Part model, mm, in its own coordinate system. Face numbers are marked on the shaded views. A direction names the side the tool comes from. Coordinates: 2 decimals unless noted, no trailing zeros. Order: outer loops, then holes, each group sorted by start corner. A loop starts at its lowest first (then second) coordinate and runs counter-clockwise, first axis right, second up.
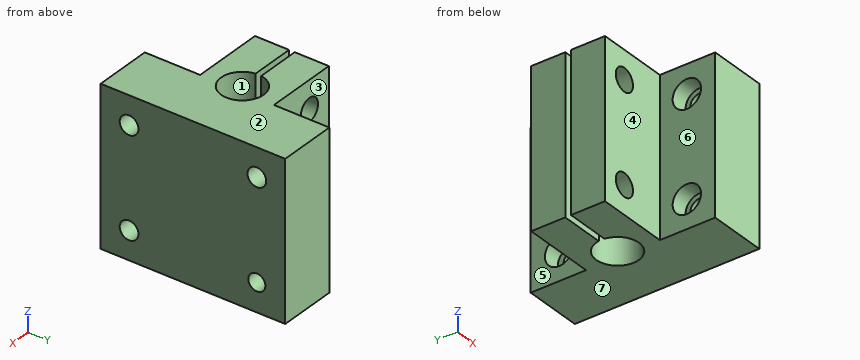
from build123d import *

# Parameters (mm, degrees)
F1_DEPTH = 55
F2_R     = 4
F3_DEPTH = 60
F4_R     = 3.3
F4_R_2   = 3
F5_DEPTH = 14.5
F6_R     = 5
F7_DEPTH = 6
F8_R     = 5
F9_DEPTH = 6


with BuildPart() as f1:
    # F0 (on Top) → F1 (new body)
    with BuildSketch(Plane.XY):
        with BuildLine():
            Line((22.920288, 15.639662), (22.920288, 25.639662))
            Line((22.920288, 25.639662), (8.420288, 25.639662))
            Line((8.420288, 25.639662), (2.420288, 25.639662))
            Line((2.420288, 25.639662), (2.420288, 6.139662))
            Line((2.420288, 6.139662), (-23.079712, 6.139662))
            Line((-23.079712, 6.139662), (-23.079712, -5.860338))
            Line((-23.079712, -5.860338), (-7.512746, -5.860338))
            ThreePointArc((-7.512746, -5.860338), (7.420288, -6.860338), (-7.512746, -7.860338))
            Line((-7.512746, -7.860338), (-23.079712, -7.860338))
            Line((-23.079712, -7.860338), (-23.079712, -19.860338))
            Line((-23.079712, -19.860338), (-0.079712, -19.860338))
            Line((-0.079712, -19.860338), (2.420288, -19.860338))
            Line((2.420288, -19.860338), (2.420288, -39.360338))
            Line((2.420288, -39.360338), (22.920288, -39.360338))
            Line((22.920288, -39.360338), (22.920288, -29.360338))
            Line((22.920288, -29.360338), (22.920288, 15.639662))
        make_face()
    extrude(amount=F1_DEPTH)

    # F2 (on face) → F3 (cut)
    with BuildSketch(Plane(origin=(0, 6.139662, 0), x_dir=(-1, 0, 0), z_dir=(0, 1, 0))):
        with Locations((14.079712, 10)):
            Circle(F2_R)
        with Locations((14.079712, 45)):
            Circle(F2_R)
    extrude(amount=-F3_DEPTH, mode=Mode.SUBTRACT)

    # F4 (on face) → F5 (cut)
    with BuildSketch(Plane.YZ.offset(22.920288)):
        with Locations((-29.360338, 10)):
            Circle(F4_R)
        with Locations((15.639662, 10)):
            Circle(F4_R_2)
        with Locations((15.639662, 45)):
            Circle(F4_R)
        with Locations((-29.360338, 45)):
            Circle(F4_R)
    extrude(amount=-F5_DEPTH, mode=Mode.SUBTRACT)

    # F6 (on face) → F7 (cut)
    with BuildSketch(Plane(origin=(2.420288, 0, 0), x_dir=(0, -1, 0), z_dir=(-1, 0, 0))):
        with Locations((29.360338, 45)):
            Circle(F6_R)
        with Locations((29.360338, 10)):
            Circle(F6_R)
    extrude(amount=-F7_DEPTH, mode=Mode.SUBTRACT)

    # F8 (on face) → F9 (cut)
    with BuildSketch(Plane(origin=(2.420288, 0, 0), x_dir=(0, -1, 0), z_dir=(-1, 0, 0))):
        with Locations((-15.639662, 45)):
            Circle(F8_R)
        with Locations((-15.639662, 10)):
            Circle(F8_R)
    extrude(amount=-F9_DEPTH, mode=Mode.SUBTRACT)


solid = f1.part
Q1. Cut at C-C on y = 2. Write the cut outline in (x, z), and give its area (3 significant figures).
Results list:
outline: (-23.08, 0) - (22.92, 0) - (22.92, 55) - (-23.08, 55) - close; hole circle Ø8 at (-14.08, 10); hole circle Ø8 at (-14.08, 45)
area: 2,430 mm2
Q2. Which spindle directions (+Z, -Z, +X, -X, +Y, -Y) get a long thin tool onto all of the face, cutting with end or side? Do the marked faces 5, 6 and 7. Say none if no direction does.
Results list:
face 5: +Z, -Z, -X, +Y
face 6: +Z, -Z, -X, -Y
face 7: -Z, +X, -X, +Y, -Y
Q3. Mould opens along Y. For the marked faces 1, 2, 3 and 4 say: pulls with the +Y half, pulls with the -Y half, needs draft (parallel to the pull), parting line crosses it, or undercut.
Results list:
face 1: undercut
face 2: needs draft
face 3: pulls with the +Y half
face 4: pulls with the -Y half
Q4. Cut at B-B on z = 20. Write the cut outline in (x, y).
Results list:
outline: (-23.08, -19.86) - (2.42, -19.86) - (2.42, -39.36) - (22.92, -39.36) - (22.92, 25.64) - (2.42, 25.64) - (2.42, 6.14) - (-23.08, 6.14) - (-23.08, -5.86) - (-7.51, -5.86) arc R7.5 cw (long way) to (-7.51, -7.86) - (-23.08, -7.86) - close
Q5. Cut at D-D on z = 45. Count the separate pieces of the cut face and the enclosed holes in it, and give its area (3 significant figures).
Results list:
separate pieces: 5
enclosed holes: 0
area: 1,280 mm2
Q6. Cut at A-A on y = -9.5. Write the cut outline in (x, z), and give its area (3 significant figures).
Results list:
outline: (-23.08, 0) - (-7.1, 0) - (-7.1, 55) - (-23.08, 55) - close; (6.94, 0) - (22.92, 0) - (22.92, 55) - (6.94, 55) - close; hole circle Ø8 at (-14.08, 10); hole circle Ø8 at (-14.08, 45)
area: 1,660 mm2
Q7. Wall check: line 1 along Z through (x, y) = (-17.5, -2); line 2 along Y through (x, z) = (2.5, 12.5); line 3 along Y through (x, z) = (-8, 4). Give the ranges that are in metal, low to high.
Results list:
line 1: z = 0 to 7.93, 12.07 to 42.93, 47.07 to 55
line 2: y = -39.36 to -33.69, -25.03 to -13.9, 0.18 to 11.31, 19.97 to 25.64
line 3: y = -19.86 to -7.86, -5.86 to 6.14
Q8. Pin check, flat tips, straight feed: pin 1 Ø10.5 at (x, z) = (-14.08, 10) entering from +Y; pin 2 Ø6.5 at (x, z) = (-14.08, 45) entering from +Y; pin 3 Ø9 at (y, z) = (15.64, 10) entering from -X; pin 4 Ø21.5 at (y, z) = (-34.5, 18.5) entering from -X. Stop position of each tip, or through.
Results list:
pin 1: stops at y = 6.14
pin 2: passes through
pin 3: stops at x = 8.42
pin 4: stops at x = 2.42
